Work out the finished part from the listing and answer in its coordinate system (mm). A direction names the side the tool comes from. Coordinates: 2 decimals unless noted, no trailing zeros. Order: outer loops, then holes, each group sorted by start corner. A loop starts at its lowest first (then second) coordinate and runs counter-clockwise, first axis right, second up.
```python
from build123d import *

# Parameters (mm, degrees)
F0_R     = 9.2
F1_DEPTH = 3
F2_DEPTH = 8
F3_W     = 7
F3_H     = 12.4
F4_DEPTH = 16
F5_DEPTH = 8
F6_R     = 1.5
F7_DEPTH = 18.501
F8_START = -5.6
F6_W     = 7
F6_H     = 4
F8_DEPTH = 6.8


with BuildPart() as f1:
    # F0 (on Top) → F1 (new body)
    with BuildSketch(Plane.XY):
        Polygon((-7.101408311, -12.3), (-14.2028166221, 0), (-7.101408311, 12.3), (-10.101408311, 12.3), (-17.2028166221, 0), (-10.101408311, -12.3), align=None)
        Polygon((-7.101408311, 12.3), (-14.2028166221, 0), (-7.101408311, -12.3), (7.101408311, -12.3), (14.2028166221, 0), (7.101408311, 12.3), align=None)
        Circle(F0_R, mode=Mode.SUBTRACT)
        Polygon((10.101408311, 12.3), (7.101408311, 12.3), (14.2028166221, 0), (7.101408311, -12.3), (10.101408311, -12.3), (17.2028166221, 0), align=None)
    extrude(amount=F1_DEPTH)

    # F0 (on Top) → F2 (join)
    with BuildSketch(Plane.XY):
        Polygon((-7.101408311, -12.3), (-14.2028166221, 0), (-7.101408311, 12.3), (-10.101408311, 12.3), (-17.2028166221, 0), (-10.101408311, -12.3), align=None)
        Polygon((10.101408311, 12.3), (7.101408311, 12.3), (14.2028166221, 0), (7.101408311, -12.3), (10.101408311, -12.3), (17.2028166221, 0), align=None)
    extrude(amount=F2_DEPTH)

    # F3 (on face) → F4 (join)
    with BuildSketch(Plane.XY.offset(8)):
        Polygon((-16.2, 1.7369293401), (-13.6232449531, 6.2), (-16.2, 6.2), align=None)
        Polygon((-14.2028166221, 0), (-10.6232449531, 6.2), (-13.6232449531, 6.2), (-16.2, 1.7369293401), (-16.2, -1.7369293401), (-13.6232449531, -6.2), (-10.6232449531, -6.2), align=None)
        Polygon((-16.2, -6.2), (-13.6232449531, -6.2), (-16.2, -1.7369293401), align=None)
        Polygon((-9.2, -6.2), (-9.2, 6.2), (-10.6232449531, 6.2), (-14.2028166221, 0), (-10.6232449531, -6.2), align=None)
        with Locations((12.7, 0)):
            Rectangle(F3_W, F3_H)
    extrude(amount=F4_DEPTH)

    # F5 (add, through all): faces of the model
    f5_faces = [f1.faces().sort_by_distance(p)[0] for p in [
        (-15.341081651, 4.71230978, 8),
        (15.341081651, 4.71230978, 8),
        (15.341081651, -4.71230978, 8),
        (-15.341081651, -4.71230978, 8),
    ]]
    extrude(f5_faces, amount=F5_DEPTH)

    # F6 (on face) → F7 (cut, through all)
    with BuildSketch(Plane.XZ.offset(6.2)):
        with Locations((-12.7, 22)):
            Circle(F6_R)
        with Locations((12.7, 22)):
            Circle(F6_R)
    extrude(amount=-F7_DEPTH, mode=Mode.SUBTRACT)

    # F6 (on face) → F8 (cut)
    with BuildSketch(Plane.XZ.offset(6.2).offset(F8_START)):
        with Locations((-12.7, 22)):
            Rectangle(F6_W, F6_H)
        with Locations((-12.7, 22)):
            Circle(F6_R, mode=Mode.SUBTRACT)
        with Locations((12.7, 22)):
            Rectangle(F6_W, F6_H)
        with Locations((12.7, 22)):
            Circle(F6_R, mode=Mode.SUBTRACT)
    extrude(amount=-F8_DEPTH, mode=Mode.SUBTRACT)


solid = f1.part
```
1. The part is cut by section C-C (y = 5). Determine the outline of the cut face in (x, z).
2. Flat-ended cylindrical pins translate along their axes: pin 1 (10 mm diameter, centred on y = -1.5, z = 19, fed in from -X); pin 2 (7.5 mm diameter, centred on x = -11, z = 14.5, fed in from +Y); pin 3 (6 mm diameter, centred on y = -4.5, z = 2.5, fed in from +X). Find the tip coordinate at first contact, or state that the pin passes through.
3. The part is cut by section B-B (z = 5.75). Determine the outline of the cut face in (x, y).
4. For faces 4 (the flat face through (-9.2, 0, 16)), 5 (the flat face through (-10.6, -6.24, 5.46)), 6 (the flat face through (-10, 9, 8)), 7 (the flat face through (-13, -6.2, 14)), determine the directions among +Z, -Z, +X, -X, +Y, -Y from which every point of the face is accessible in a straight line to the end or side of a thin tool.
5. The part is cut by section D-D (x = -12.7). Determine the outline of the cut face in (y, z).
6. Consider probe 1 along Z at (x, y) = (-12.7, -2.4); probe 2 along X at (y, z) = (0, 5.75); probe 3 along X at (y, z) = (4.5, 13.5). Determine where each line is inside the solid, lowest interval first.
7. The part is cut by section A-A (x = 0). Determine the outline of the cut face in (y, z), plus the area to 3 significant figures.
8. The mould has two halves that part along Z. Classify faces 1 (the flat face through (-13, -3, 24)), 2 (the flat face through (0, 12.3, 2)), 3 (the flat face through (-11, 0, 8)): released by +Z, released by -Z, zero draft, split by the parting line, or undercut.
Worked out:
1. outline: (-16.2, 0) - (-7.72, 0) - (-7.72, 3) - (-11.32, 3) - (-11.32, 8) - (-9.2, 8) - (-9.2, 20) - (-16.2, 20) - close; (7.72, 0) - (16.2, 0) - (16.2, 20) - (9.2, 20) - (9.2, 8) - (11.32, 8) - (11.32, 3) - (7.72, 3) - close
2. pin 1: stops at x = -16.2
2. pin 2: stops at y = 6.2
2. pin 3: stops at x = 16.34
3. outline: (-17.2, 0) - (-16.2, -1.74) - (-16.2, -6.2) - (-13.62, -6.2) - (-10.1, -12.3) - (-7.1, -12.3) - (-14.2, 0) - (-7.1, 12.3) - (-10.1, 12.3) - (-13.62, 6.2) - (-16.2, 6.2) - (-16.2, 1.74) - close; (7.1, -12.3) - (10.1, -12.3) - (13.62, -6.2) - (16.2, -6.2) - (16.2, -1.74) - (17.2, 0) - (16.2, 1.74) - (16.2, 6.2) - (13.62, 6.2) - (10.1, 12.3) - (7.1, 12.3) - (14.2, 0) - close
4. face 4: +Z, +Y, -Y
4. face 5: none
4. face 6: +Z, +X, -X, +Y
4. face 7: +Z, -X, -Y
5. outline: (-7.8, 0) - (7.8, 0) - (7.8, 8) - (6.2, 8) - (6.2, 20) - (-0.6, 20) - (-0.6, 20.5) - (-6.2, 20.5) - (-6.2, 8) - (-7.8, 8) - close; (-6.2, 23.5) - (-0.6, 23.5) - (-0.6, 24) - (-6.2, 24) - close; hole (-2.6, 3) - (2.6, 3) - (2.6, 8) - (-2.6, 8) - close
6. probe 1: z = 0 to 3, 8 to 20.5, 23.5 to 24
6. probe 2: x = -17.2 to -14.2, 14.2 to 17.2
6. probe 3: x = -16.2 to -9.2, 9.2 to 16.2
7. outline: (-12.3, 0) - (-9.2, 0) - (-9.2, 3) - (-12.3, 3) - close; (9.2, 0) - (12.3, 0) - (12.3, 3) - (9.2, 3) - close
7. area: 18.6 mm2
8. face 1: released by +Z
8. face 2: zero draft
8. face 3: undercut
